Here's how the part is built. I have some questions about the finished solid (model axes, mm). A direction names the side the tool comes from. Coordinates: 2 decimals unless noted, no trailing zeros. Write each loop counter-clockwise with the first axis right and the second up, starting at its lowest first coordinate (ties: lowest second). Pieces come first, ordered by that corner, then holes.
Item 1: We'd pull the mould along Y, two halves only. Please class faces 6 (the face through (2.285, 3.584, -30.472)), 7 (the face through (-25, 42, -27)), 8 (the face through (-39, -20, -32)), 9 (the face through (20, 23, -30)): +Y half, -Y half, draft (parallel to the pull), parting line (faces both ways), or undercut.
Item 2: For faces 1 (the face through (2.828, 54.923, -30.472)), 2 (the face through (-65, 72.5, -33)), 3 (the face through (-49, 34, -23)), 4 (the face through (-40.79, 27.23, -32.94)), 5 (the face through (-12.9, 63, -30.5)), which set-ups out of +Z, -Z, +X, -X, +Y, -Y let a thin tool reach every point of the face, with its end or its side?
Item 3: If I drill on line 1 (Y direction, x = -35.5, z = -30.75); line 2 (Z direction, x = -4.5, y = 50.5); line 3 (X direction, y = 50, z = -34.75), over which ranges is the centre line in solid material (lowest first)?
Item 4: If we section it at C-C (x = -56): Please give me the cut outline in (y, z), then the cut area to 3 significant figures.
Item 5: If we section it at B-B (z = -22.5): Please give me the cut outline in (x, y), then the cut area to 3 significant figures.
Item 6: I'm going to push flat-ended pins straight in: pin 1 Ø8 at (x, y) = (-50, -10) entering from +Z; pin 2 Ø1.5 at (y, z) = (31.5, -29) entering from +X; pin 3 Ø3 at (x, z) = (-0.5, -31) entering from +Y. Where does each tip first touch, or does it pass through?
Item 7: If we section it at A-A (y = 60.5): Please give me the cut outline in (x, z).
Item 8: If we section it at D-D (x = 0): Please give me the cut outline in (y, z).
from build123d import *

# Parameters (mm, degrees)
SKETCH023_R       = 4.25
SKETCH023_R_2     = 9
SKETCH023_W       = 6
SKETCH023_H       = 3
PAD013_DEPTH      = 8
PAD013_DEPTH_BACK = 9
POCKET010_DEPTH   = 5.001
SKETCH028_R       = 17
POCKET011_DEPTH   = 6.501
POCKET012_DEPTH   = 8.001
POCKET013_DEPTH   = 5.001
SKETCH031_R       = 9
PAD014_DEPTH      = 4
POCKET014_DEPTH   = 9.001


with BuildPart() as part:
    # Sketch023 → Pad013 (new body, two sides)
    with BuildSketch(Plane.XY) as pad013_sk:
        with BuildLine():
            Line((20, 58), (20, -13))
            ThreePointArc((13, -20), (17.949747, -17.949747), (20, -13))
            Line((13, -20), (-73, -20))
            ThreePointArc((-80, -13), (-77.949747, -17.949747), (-73, -20))
            Line((-80, -13), (-80, 71))
            ThreePointArc((-73, 78), (-77.949747, 75.949747), (-80, 71))
            Line((-73, 78), (-18, 78))
            Line((-18, 35), (-18, 78))
            Line((-33, 32), (-18, 35))
            Line((-73, 32), (-33, 32))
            ThreePointArc((-73, 32), (-74.767767, 31.267767), (-75.5, 29.5))
            Line((-75.5, 29.5), (-75.5, -13))
            ThreePointArc((-75.5, -13), (-73.751764, -15.384292), (-70.95212, -14.433941))
            Line((-70.95212, -14.433941), (-43.329649, 25.015035))
            ThreePointArc((-37.595585, 28), (-40.827825, 27.209076), (-43.329649, 25.015035))
            Line((-37.595585, 28), (-22, 28))
            ThreePointArc((-22, 28), (-17.050253, 30.050253), (-15, 35))
            Line((-15, 35), (-15, 58))
            ThreePointArc((-8, 65), (-12.949747, 62.949747), (-15, 58))
            Line((-8, 65), (13, 65))
            ThreePointArc((20, 58), (17.949747, 62.949747), (13, 65))
        make_face()
        Circle(SKETCH023_R, mode=Mode.SUBTRACT)
        with Locations((4, 46)):
            Circle(SKETCH023_R_2, mode=Mode.SUBTRACT)
        with BuildLine():
            ThreePointArc((-38, 63), (-47, 54), (-38, 45))
            Line((-38, 45), (-35, 45))
            ThreePointArc((-35, 45), (-26, 54), (-35, 63))
            Line((-35, 63), (-38, 63))
        make_face(mode=Mode.SUBTRACT)
        with BuildLine():
            ThreePointArc((-67, 70), (-69, 68), (-67, 66))
            Line((-67, 66), (-64, 66))
            ThreePointArc((-64, 66), (-62, 68), (-64, 70))
            Line((-64, 70), (-67, 70))
        make_face(mode=Mode.SUBTRACT)
        with BuildLine():
            ThreePointArc((-67, 42), (-69, 40), (-67, 38))
            Line((-67, 38), (-64, 38))
            ThreePointArc((-64, 38), (-62, 40), (-64, 42))
            Line((-64, 42), (-67, 42))
        make_face(mode=Mode.SUBTRACT)
        with Locations((6, 34.5)):
            Rectangle(SKETCH023_W, SKETCH023_H, mode=Mode.SUBTRACT)
        with Locations((-6, 34.5)):
            Rectangle(SKETCH023_W, SKETCH023_H, mode=Mode.SUBTRACT)
        with BuildLine():
            ThreePointArc((-27, 70), (-29, 68), (-27, 66))
            Line((-27, 66), (-24, 66))
            ThreePointArc((-24, 66), (-22, 68), (-24, 70))
            Line((-24, 70), (-27, 70))
        make_face(mode=Mode.SUBTRACT)
        with BuildLine():
            ThreePointArc((-27, 42), (-29, 40), (-27, 38))
            Line((-27, 38), (-24, 38))
            ThreePointArc((-24, 38), (-22, 40), (-24, 42))
            Line((-24, 42), (-27, 42))
        make_face(mode=Mode.SUBTRACT)
    extrude(amount=PAD013_DEPTH)
    extrude(pad013_sk.sketch, amount=-PAD013_DEPTH_BACK)

    # Sketch025 → Pocket010 (cut, through all)
    with BuildSketch(Plane.XY.offset(3)):
        Polygon((-76.145312, 74), (-16.940075, 74), (-16.940075, 34), (-76, 34), align=None)
    extrude(amount=POCKET010_DEPTH, mode=Mode.SUBTRACT)

    # Sketch028 → Pocket011 (cut, through all)
    with BuildSketch(Plane.YZ.offset(-73.5)):
        with Locations((53.5, 14)):
            Circle(SKETCH028_R)
    extrude(amount=-POCKET011_DEPTH, mode=Mode.SUBTRACT)

    # Sketch029 → Pocket012 (cut, through all)
    with BuildSketch(Plane.XY):
        Polygon((-85.091896, 32), (-85.091896, -28.781052), (33.933025, -28.781052), (33.933025, 68.141579), (-16, 68.141579), (-16, 32), align=None)
    extrude(amount=POCKET012_DEPTH, mode=Mode.SUBTRACT)

    # Sketch030 → Pocket013 (cut, through all)
    with BuildSketch(Plane.XY.offset(-4)):
        Polygon((30.837446, 73.192078), (-15.70892, 73.192078), (-15.70892, 34.728077), (-25, 32), (-25, -27.823572), (30.837446, -27.823572), align=None)
    extrude(amount=-POCKET013_DEPTH, mode=Mode.SUBTRACT)

    # Sketch031 → Pad014 (join)
    with BuildSketch(Plane.XY.offset(-5)):
        with BuildLine():
            ThreePointArc((-12.961917, 32.170317), (21.901003, 28.600337), (15.969569, 63.139967))
            Line((-7.855077, 75.521284), (15.969569, 63.139967))
            ThreePointArc((-7.855077, 75.521284), (-12.778326, 77.371339), (-18, 78))
            Line((-18, 78), (-18, 35))
            ThreePointArc((-12.961917, 32.170317), (-15.110823, 34.244164), (-18, 35))
        make_face()
        with Locations((5.824645, 43.618683)):
            Circle(SKETCH031_R, mode=Mode.SUBTRACT)
    extrude(amount=-PAD014_DEPTH)

    # Sketch032 → Pocket014 (cut, through all)
    with BuildSketch(Plane.XY):
        with BuildLine():
            ThreePointArc((-67, 44.5), (-71.5, 40), (-67, 35.5))
            Line((-67, 35.5), (-64, 35.5))
            ThreePointArc((-64, 35.5), (-59.5, 40), (-64, 44.5))
            Line((-64, 44.5), (-67, 44.5))
        make_face()
        with BuildLine():
            ThreePointArc((-67, 72.5), (-71.5, 68), (-67, 63.5))
            Line((-67, 63.5), (-64, 63.5))
            ThreePointArc((-64, 63.5), (-59.5, 68), (-64, 72.5))
            Line((-64, 72.5), (-67, 72.5))
        make_face()
        with BuildLine():
            ThreePointArc((-27, 72.5), (-31.5, 68), (-27, 63.5))
            Line((-27, 63.5), (-24, 63.5))
            ThreePointArc((-24, 63.5), (-19.5, 68), (-24, 72.5))
            Line((-24, 72.5), (-27, 72.5))
        make_face()
        with BuildLine():
            ThreePointArc((-27, 44.5), (-31.5, 40), (-27, 35.5))
            Line((-27, 35.5), (-24, 35.5))
            ThreePointArc((-24, 35.5), (-19.5, 40), (-24, 44.5))
            Line((-24, 44.5), (-27, 44.5))
        make_face()
    extrude(amount=-POCKET014_DEPTH, mode=Mode.SUBTRACT)


with BuildPart() as part_1:
    # Body009 placement: moved
    add(part.part.moved(Location((0, 0, -28.5))))


solid = part_1.part
Answer list:
1. face 6: undercut
1. face 7: undercut
1. face 8: -Y half
1. face 9: draft
2. face 1: +Z
2. face 2: -Z
2. face 3: +Z, +X
2. face 4: +Z, -Z
2. face 5: +Z, +Y
3. line 1: y = -20 to 28, 32 to 45, 63 to 78
3. line 2: z = -37.5 to -33.5, -32.5 to -28.5
3. line 3: x = -80 to -46.06, -26.94 to -0.52, 12.17 to 26.88
4. outline: (-20, -37.5) - (6.92, -37.5) - (6.92, -28.5) - (-20, -28.5) - close; (32, -37.5) - (78, -37.5) - (78, -20.5) - (74, -20.5) - (74, -25.5) - (34, -25.5) - (34, -20.5) - (32, -20.5) - close
4. area: 824 mm2
5. outline: (-80, 32) - (-33, 32) - (-23, 34) - (-76, 34) - (-76.02, 38.5) - (-80, 38.5) - close; (-80, 68.5) - (-76.13, 68.5) - (-76.15, 74) - (-18, 74) - (-18, 78) - (-73, 78) arc R7 ccw to (-80, 71) - close
5. area: 381 mm2
6. pin 1: stops at z = -28.5
6. pin 2: stops at x = 20
6. pin 3: stops at y = 65
7. outline: (-80, -37.5) - (-44.22, -37.5) - (-44.22, -25.5) - (-73.5, -25.5) - (-73.5, -29.99) - (-80, -29.99) - close; (-28.78, -37.5) - (19.93, -37.5) - (19.93, -33.5) - (-18, -33.5) - (-18, -25.5) - (-28.78, -25.5) - close; (-14.54, -32.5) - (19.54, -32.5) - (19.54, -28.5) - (-14.54, -28.5) - close
8. outline: (-20, -32.5) - (-4.25, -32.5) - (-4.25, -28.5) - (-20, -28.5) - close; (4.25, -32.5) - (37.94, -32.5) - (37.94, -28.5) - (4.25, -28.5) - close; (22.4, -37.5) - (36.76, -37.5) - (36.76, -33.5) - (22.4, -33.5) - close; (50.48, -37.5) - (71.44, -37.5) - (71.44, -33.5) - (50.48, -33.5) - close; (54.06, -32.5) - (65, -32.5) - (65, -28.5) - (54.06, -28.5) - close
